from build123d import *

# Parameters (mm, degrees)
SALIENTE_EXTRUIR1_DEPTH = 3
CROQUIS2_W              = 380
CROQUIS2_H              = 160
CORTAR_EXTRUIR1_DEPTH   = 3


with BuildPart() as part:
    # Croquis1 → Saliente-Extruir1 (new body)
    with BuildSketch(Plane(origin=(0, 0, 0), x_dir=(1, 0, 0), z_dir=(0, 1, 0))):
        Polygon((480, 280), (480, 283.1), (460, 283.1), (460, 280), (440, 280), (440, 283.1), (420, 283.1), (420, 280), (400, 280), (400, 283.1), (380, 283.1), (380, 280), (360, 280), (360, 283.1), (340, 283.1), (340, 280), (320, 280), (320, 283.1), (300, 283.1), (300, 280), (280, 280), (280, 283.1), (260, 283.1), (260, 280), (240, 280), (240, 283.1), (220, 283.1), (220, 280), (200, 280), (200, 283.1), (180, 283.1), (180, 280), (160, 280), (160, 283.1), (140, 283.1), (140, 280), (120, 280), (120, 283.1), (100, 283.1), (100, 280), (80, 280), (80, 283.1), (60, 283.1), (60, 280), (40, 280), (40, 283.1), (20, 283.1), (20, 280), (0, 280), (0, 260), (-3.1, 260), (-3.1, 240), (0, 240), (0, 220), (-3.1, 220), (-3.1, 200), (0, 200), (0, 180), (-3.1, 180), (-3.1, 160), (0, 160), (0, 140), (-3.1, 140), (-3.1, 120), (0, 120), (0, 100), (-3.1, 100), (-3.1, 80), (0, 80), (0, 60), (-3.1, 60), (-3.1, 40), (0, 40), (0, 20), (-3.1, 20), (-3.1, 0), (0, 0), (480, 0), (480, 20), (483.1, 20), (483.1, 40), (480, 40), (480, 60), (483.1, 60), (483.1, 80), (480, 80), (480, 100), (483.1, 100), (483.1, 120), (480, 120), (480, 140), (483.1, 140), (483.1, 160), (480, 160), (480, 180), (483.1, 180), (483.1, 200), (480, 200), (480, 220), (483.1, 220), (483.1, 240), (480, 240), (480, 260), (483.1, 260), (483.1, 280), align=None)
    extrude(amount=SALIENTE_EXTRUIR1_DEPTH)

    # Croquis2 → Cortar-Extruir1 (cut)
    with BuildSketch(Plane(origin=(0, 3, 0), x_dir=(1, 0, 0), z_dir=(0, 1, 0))):
        with Locations((240, 150)):
            Rectangle(CROQUIS2_W, CROQUIS2_H)
    extrude(amount=-CORTAR_EXTRUIR1_DEPTH, mode=Mode.SUBTRACT)


solid = part.part
Geometry check sheet. Reference: the model listing, model coordinates, mm. Round coordinates to 2 decimals unless told otherwise and drop trailing zeros. Write each loop counter-clockwise with the first axis right and the second up, starting at its lowest first coordinate (ties: lowest second). Pieces come first, ordered by that corner, then holes. Notation, with made-up numbers: (32, 0) - (82, 0) arc R24 cw to (82, 23) - close; hole circle Ø2 at (41.25, 45.5). An arc over 180 degrees is marked (long way). One line per item, written item: value.
1. Depth check by flat-ended pin: pin 1 Ø0.9 at (x, y) = (408, 1.5) entering from -Z; pin 2 Ø1.5 at (y, z) = (1.5, -86.5) entering from +X; pin 3 Ø1.5 at (x, y) = (-2, 1.5) entering from +Z. Enter the tip coordinate at first touch or a pass-through.
The answers:
pin 1: stops at z = -280
pin 2: stops at x = 480
pin 3: stops at z = 0
2. Scan lines: L1, parallel to X at y = 2.4, z = -221.5; L2, parallel to Z at x = 394.5, y = 2.6; L3, parallel to X at y = 1.65, z = -91. Record each from-to range of solid material in increasing order.
The answers:
L1: x = 0 to 50, 430 to 483.1
L2: z = -283.1 to -230, -70 to 0
L3: x = -3.1 to 50, 430 to 480
3. Cross-section at A-A on z = -115. Record the boundary of the cut face in (x, y), and give its area (3 significant figures).
The answers:
outline: (0, 0) - (50, 0) - (50, 3) - (0, 3) - close; (430, 0) - (483.1, 0) - (483.1, 3) - (430, 3) - close
area: 309 mm^2
4. Cross-section at B-B on x = 305. Record the boundary of the cut face in (y, z), and give its area (3 significant figures).
The answers:
outline: (0, -283.1) - (3, -283.1) - (3, -230) - (0, -230) - close; (0, -70) - (3, -70) - (3, 0) - (0, 0) - close
area: 369 mm^2
